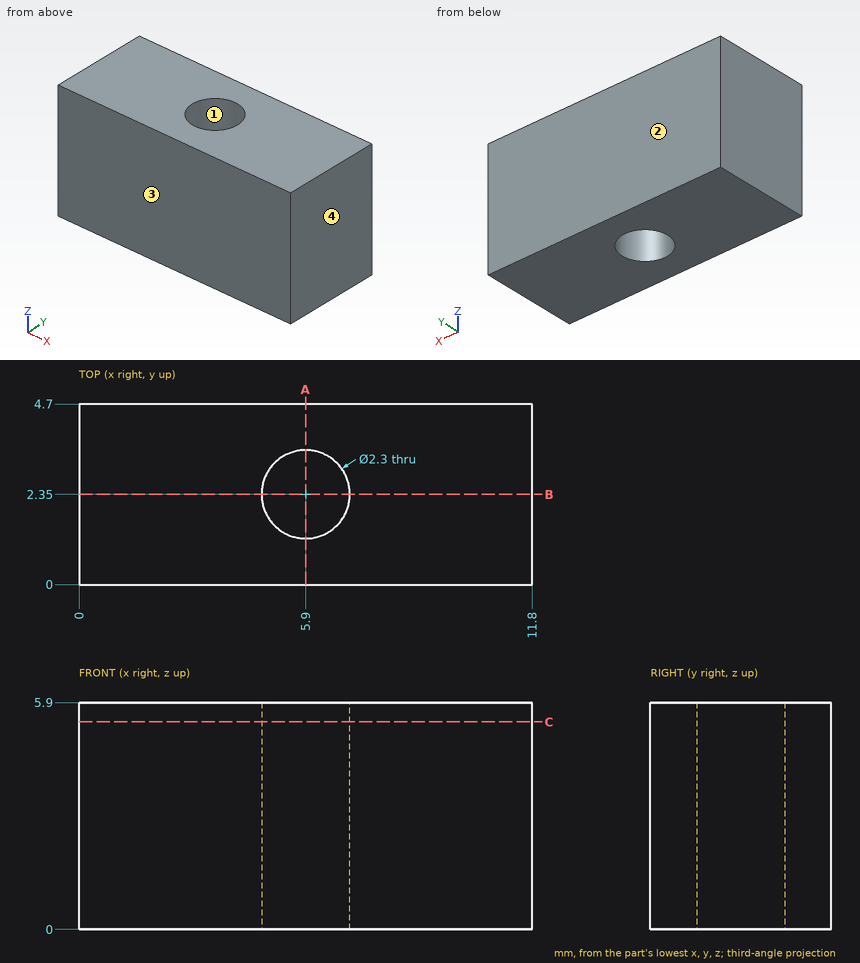
Could you check a few things on this drawing? It's one solid part, dimensions in mm from its lowest x, y, z. Round coordinates to 2 decimals unless told otherwise and drop trailing zeros. Loops run counter-clockwise (first coordinate to the right, second up) from the corner with the lowest first, then second, coordinate; pieces in that order, holes last.
Q1. Please list where these lines run through material, in increasing order: L1, parallel to Y at x = 5.9, z = 1.6; L2, parallel to X at y = 1.5, z = 2.8; L3, parallel to Y at x = 6.25, z = 1.2.
Q2. I want a section at C-C (z = 5.4). Write out the boundary of the cut face in (x, y), and give its area (3 significant figures).
Q3. Thinking about a two-plate mould opening in Y: for the marked faces 1, 2, 3 and 4, which applies, pulls with the +Y half, pulls with the -Y half, needs draft (parallel to the pull), parting line crosses it, or undercut?
Q4. I want a section at B-B (y = 2.35). Write out the boundary of the cut face in (x, z).
Q5. I want a section at A-A (x = 5.9). Write out the boundary of the cut face in (y, z), and give its area (3 significant figures).
Answer below:
1. L1: y = 0 to 1.2, 3.5 to 4.7
1. L2: x = 0 to 5.13, 6.67 to 11.8
1. L3: y = 0 to 1.25, 3.45 to 4.7
2. outline: (0, 0) - (11.8, 0) - (11.8, 4.7) - (0, 4.7) - close; hole circle Ø2.3 at (5.9, 2.35)
2. area: 51.3 mm2
3. face 1: undercut
3. face 2: pulls with the +Y half
3. face 3: pulls with the -Y half
3. face 4: needs draft
4. outline: (0, 0) - (4.75, 0) - (4.75, 5.9) - (0, 5.9) - close; (7.05, 0) - (11.8, 0) - (11.8, 5.9) - (7.05, 5.9) - close
5. outline: (0, 0) - (1.2, 0) - (1.2, 5.9) - (0, 5.9) - close; (3.5, 0) - (4.7, 0) - (4.7, 5.9) - (3.5, 5.9) - close
5. area: 14.2 mm2
